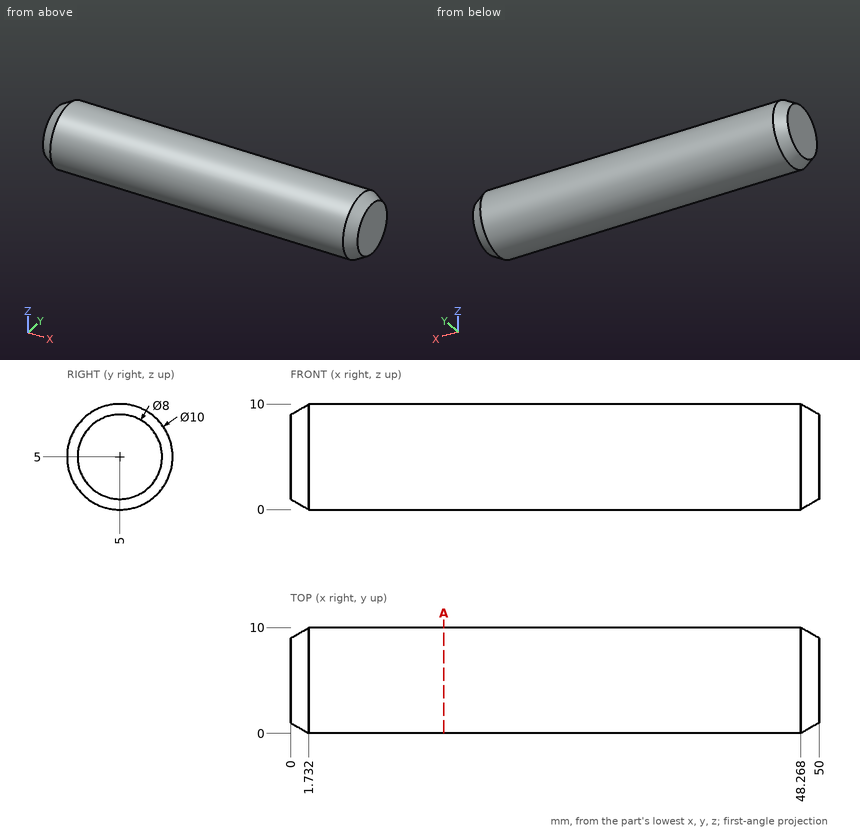
Answer from the drawing. Dimensions are ordinates in mm from the lowest x, y and z of the part. Round coordinates to 2 decimals unless told otherwise and drop trailing zeros. Write each loop counter-clockwise with the first axis right and the second up, starting at its lowest first coordinate (ties: lowest second). Pieces come first, ordered by that corner, then holes. Notation, with made-up numbers: (80.5, -19.75) -> (107.5, -19.75) arc R33 ccw to (107.5, 13.25) -> close; hole circle Ø3 at (72, 54.5). An arc over 180 degrees is marked (long way). Answer in a Markdown table with one row per item. Add a question column.
1) Consider line 1 (Y direction, x = 24.5, z = 4.75); line 2 (X direction, y = 9.5, z = 3); line 3 (Y direction, x = 11, z = 3.25). Determine where each line is inside the solid, lowest interval first.
2) Given P1, Ø4, axis at x = 19.5, y = 7.5, coming from the +Z side (3 decimals); P2, Ø1.5, axis at x = 24.5, z = 1.5, coming from the +Y side; P3, Ø1.5, axis at x = 15, z = 2, coming from the +Y side (3 decimals); P4, Ø4, axis at x = 18, z = 6, coming from the -Y side, each flat-ended and moving along its own axis, determine where each tip first touches the part or whether it passes through.
3) Find section A-A, the plane x = 14.5. Determine the outline of the cut face in (y, z), and give its area (3 significant figures).
Findings below:
| question | item | result |
|---|---|---|
| 1 | line 1 | 0.01 to 9.99 |
| 1 | line 2 | 1.6 to 48.4 |
| 1 | line 3 | 0.32 to 9.68 |
| 2 | P1 | z = 9.975 |
| 2 | P2 | y = 9.18 |
| 2 | P3 | y = 9.465 |
| 2 | P4 | y = 0 |
| 3 | outline | circle Ø10 at (5, 5) |
| 3 | area | 78.5 mm² |
